Work out the finished part from the listing and answer in its coordinate system (mm). Face numbers are marked on the shaded views. Give positions to 0.01 mm unless a question says otherwise; leave off trailing zeros. Order: outer loops, then holes, each group sorted by start corner. A loop starts at its lowest first (then second) coordinate and runs counter-clockwise, first axis right, second up. Notation, with made-up numbers: M -22.5,50.25 L 17.5,50.25 A36 cw 17.5,88.25 Z; hole C 37.25,1 d10. An arc over 180 degrees is marked long. One line per item, written item: value.
from build123d import *

# Parameters (mm, degrees)
F1_DEPTH = 6.35
F2_R     = 3.5179
F3_DEPTH = 15.876
F4_R     = 1.524
F5_R     = 3.556
F6_DEPTH = 6.35
F8_DEPTH = 1.524


# Not quite as in the source:
# - a pattern or mirror of a feature is missing from the dataset's text; its kind, count and spacing are read off the source's solid


with BuildPart() as f1:
    # F0 (on Top) → F1 (new body)
    with BuildSketch(Plane.XY):
        Polygon((0, 0), (-31.75, 0), (-31.75, -15.875), (0, -15.875), (31.75, -15.875), (31.75, 0), align=None)
    extrude(amount=F1_DEPTH)

    # F2 (on face) → F3 (cut, through all)
    with BuildSketch(Plane(origin=(0, 0, 0), x_dir=(-1, 0, 0), z_dir=(0, 1, 0))):
        with Locations((-22.733, 6.731)):
            Circle(F2_R)
        with Locations((22.733, 6.731)):
            Circle(F2_R)
    extrude(amount=-F3_DEPTH, mode=Mode.SUBTRACT)

    # F4
    f4_edges = [f1.edges().sort_by_distance(p)[0] for p in [
        (31.75, 0, 3.175),
        (31.75, -15.875, 3.175),
        (-31.75, 0, 3.175),
        (-31.75, -15.875, 3.175),
        (19.235793, -7.9375, 6.35),
        (26.230207, -7.9375, 6.35),
        (-26.230207, -7.9375, 6.35),
        (-19.235793, -7.9375, 6.35),
    ]]
    fillet(f4_edges, radius=F4_R)

    # F5 (on face) → F6 (cut, through all)
    with BuildSketch(Plane(origin=(0, 0, 0), x_dir=(1, 0, 0), z_dir=(0, 0, -1))):
        with Locations((-9.525, 7.9375)):
            Circle(F5_R)
    f6 = extrude(amount=-F6_DEPTH, mode=Mode.SUBTRACT)

    # F6_copies: F6 across plane
    add(f6.mirror(Plane(origin=(0, 0, 0), x_dir=(0, 0, 1), z_dir=(1, 0, 0))), mode=Mode.SUBTRACT)

    # F7 (on face) → F8 (cut)
    with BuildSketch(Plane(origin=(0, 0, 0), x_dir=(1, 0, 0), z_dir=(0, 0, -1))):
        Polygon((-9.525, 1.984375), (-6.0879616787, 1.984375), (-2.6509233575, 7.9375), (-6.0879616787, 13.890625), (-9.525, 13.890625), (-12.9620383213, 13.890625), (-16.3990766425, 7.9375), (-12.9620383213, 1.984375), align=None)
    f8 = extrude(amount=-F8_DEPTH, mode=Mode.SUBTRACT)

    # F8_copies: F8 across plane
    add(f8.mirror(Plane(origin=(0, 0, 0), x_dir=(0, 0, 1), z_dir=(1, 0, 0))), mode=Mode.SUBTRACT)


solid = f1.part
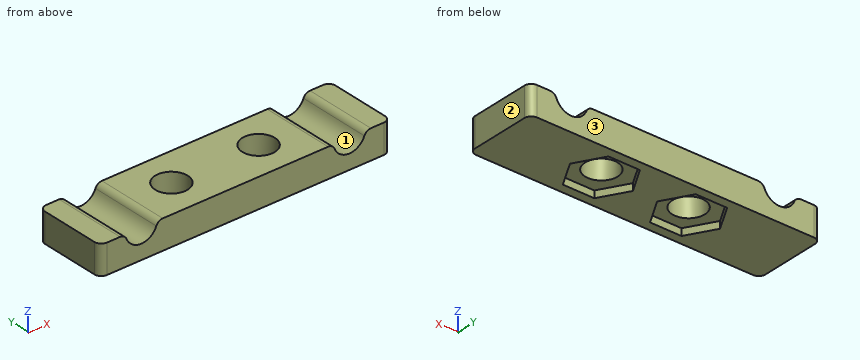
(1) Find the intervals of material crossed by probe 1 along X at (y, z) = (-6, 0.75); probe 2 along Y at (x, z) = (-9.5, 5.75) (3 decimals); probe 3 along X at (y, z) = (-4, 3.5), in increasing order. Write a range as from..to.
Findings:
probe 1: x = -31.75..-15.28, -3.77..3.77, 15.28..31.75
probe 2: y = -15.875..-11.493, -4.382..0
probe 3: x = -31.75..-24.12, -21.34..21.34, 24.12..31.75
(2) Section A-A, the plane z = 4 is taken. Give the number of separate pieces and of enclosed holes in the cut face, then the cut area to 3 significant figures.
Findings:
separate pieces: 3
enclosed holes: 2
area: 786 mm^2
(3) Section C-C, the plane y = -6 is taken. Give the vertices of the cut face in (x, z).
Findings:
outline: M -31.75,0 L -15.28,0 L -15.28,1.52 L -12.51,1.52 L -12.51,6.35 L -18.06,6.35 A1.52 ccw -19.48,5.4 A3.52 cw -25.99,5.4 A1.52 ccw -27.4,6.35 L -31.75,6.35 Z; M -6.54,1.52 L -3.77,1.52 L -3.77,0 L 3.77,0 L 3.77,1.52 L 6.54,1.52 L 6.54,6.35 L -6.54,6.35 Z; M 12.51,1.52 L 15.28,1.52 L 15.28,0 L 31.75,0 L 31.75,6.35 L 27.4,6.35 A1.52 ccw 25.99,5.4 A3.52 cw 19.48,5.4 A1.52 ccw 18.06,6.35 L 12.51,6.35 Z
(4) Section D-D, the plane x = 3.5 is taken. Give the vertices of the cut face in (y, z) (3 decimals), then the cut area to 3 significant figures.
Findings:
outline: M -15.875,0 L -9.408,0 L -9.408,1.524 L -6.467,1.524 L -6.467,0 L 0,0 L 0,6.35 L -15.875,6.35 Z
area: 96.3 mm^2
(5) Determine the mould class of the marked faces 1, 2 and 3 for opening direction X: pulls with the +X half, pulls with the -X half, needs draft (parallel to the pull), parting line crosses it, or undercut.
Findings:
face 1: undercut
face 2: pulls with the +X half
face 3: needs draft
(6) Section B-B, the plane x = 10 is taken. Give the vertices of the cut face in (y, z) (3 decimals), then the cut area to 3 significant figures.
Findings:
outline: M -15.875,0 L -13.891,0 L -13.891,1.524 L -11.462,1.524 L -11.462,6.35 L -15.875,6.35 Z; M -4.413,1.524 L -1.984,1.524 L -1.984,0 L 0,0 L 0,6.35 L -4.413,6.35 Z
area: 48.6 mm^2
(7) Given P1, Ø6.5, axis at x = -9.52, y = -7.94, coming from the +Z side, flat-ended and moving along its own axis, determine where the tip first touches the part or whether it passes through.
Findings:
P1: passes through
